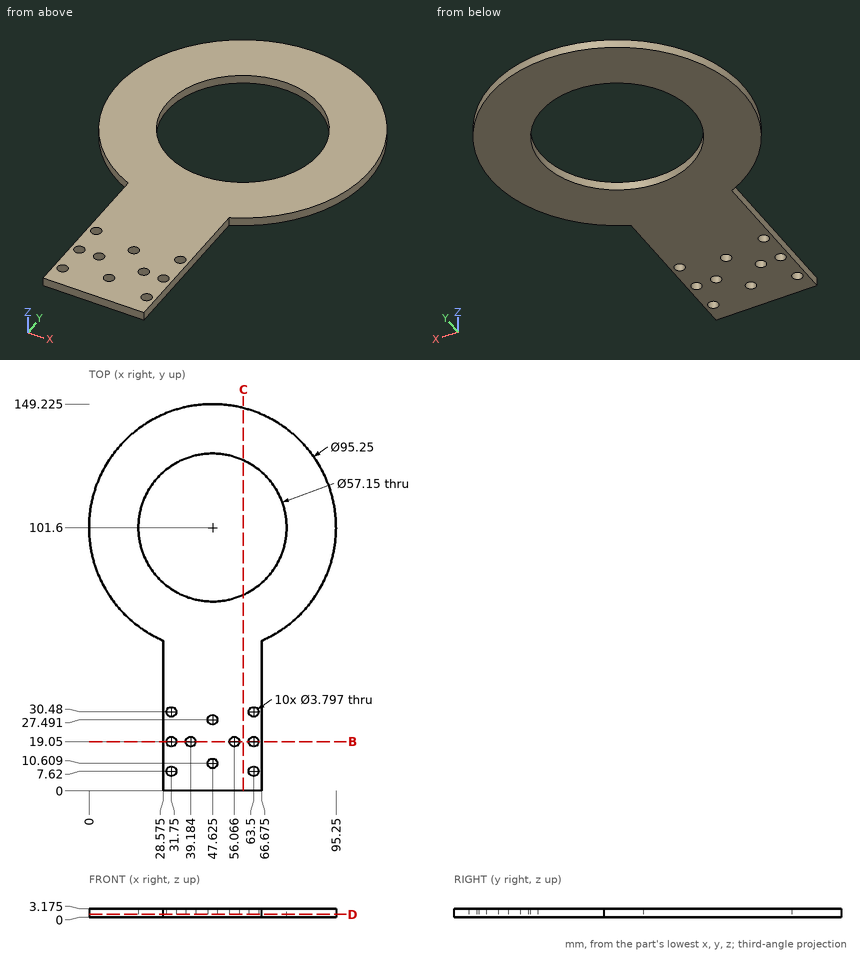
Design review of the part shown in the three views and the two pictorial views. Dimensions are in mm from the part's minimum x, y and z. Round coordinates to 2 decimals unless told otherwise and drop trailing zeros. Write each loop counter-clockwise with the first axis right and the second up, starting at its lowest first coordinate (ties: lowest second). Pieces come first, ordered by that corner, then holes. Notation, with made-up numbers: (79.25, 61) - (132.25, 61) arc R20 ccw to (132.25, 73) - close; hole circle Ø10 at (62.5, 57). An arc over 180 degrees is marked (long way). Write item = value, one per line. Start each with the question number.
1. Wall thickness on L1, parallel to X at y = 30.48, z = 1.6 (1 decimal); L2, parallel to X at y = 19.05, z = 0.8 (1 decimal); L3, parallel to Y at x = 64.5, z = 0.8 (1 decimal): over which ranges is each line inside the solid? List them lowest first.
2. Consider section C-C on x = 59.5. State the section outline as (y, z) points (1 decimal).
3. Consider section D-D on z = 1.05. Give the number of separate pieces and of enclosed holes in the cut face, plus the area to 3 significant figures.
4. For pin 1 Ø2.5 at (x, y) = (63.5, 19.05) entering from -Z; pin 2 Ø1 at (y, z) = (22, 2.5) entering from +X (3 decimals), all flat-tipped, find the tip position at first contact; note any pin that passes through.
5. Consider section B-B on y = 19.05. State the section outline as (x, z) points (1 decimal).
Evaluation:
q1.L1 = 28.6 to 29.9, 33.6 to 61.6, 65.4 to 66.7
q1.L2 = 28.6 to 29.9, 33.6 to 37.3, 41.1 to 54.2, 58 to 61.6, 65.4 to 66.7
q1.L3 = 0 to 6, 9.2 to 17.4, 20.7 to 28.9, 32.1 to 78.5, 124.7 to 146.1
q2.outline = (0, 0) - (75.6, 0) - (75.6, 3.2) - (0, 3.2) - close; (127.6, 0) - (147.7, 0) - (147.7, 3.2) - (127.6, 3.2) - close
q3.separate_pieces = 1
q3.enclosed_holes = 11
q3.area = 6,550 mm2
q4.pin_1 = through
q4.pin_2 = 66.675
q5.outline = (28.6, 0) - (29.9, 0) - (29.9, 3.2) - (28.6, 3.2) - close; (33.6, 0) - (37.3, 0) - (37.3, 3.2) - (33.6, 3.2) - close; (41.1, 0) - (54.2, 0) - (54.2, 3.2) - (41.1, 3.2) - close; (58, 0) - (61.6, 0) - (61.6, 3.2) - (58, 3.2) - close; (65.4, 0) - (66.7, 0) - (66.7, 3.2) - (65.4, 3.2) - close
